from build123d import *

# Parameters (mm, degrees)
F0_W      = 228.6
F0_H      = 114.3
F1_DEPTH  = 120.65
F6_R      = 9.525
F7_DEPTH  = 38.1
F8_DEPTH  = 12.7
F10_DEPTH = 228.6
F11_R     = 9.525
F12_DEPTH = 31.75


# Not quite as in the source:
# - a pattern or mirror of a feature is missing from the dataset's text; its kind, count and spacing are read off the source's solid


with BuildPart() as f1:
    # F0 (on Top) → F1 (new body)
    with BuildSketch(Plane.XY):
        with Locations((-114.3, 57.15)):
            Rectangle(F0_W, F0_H)
    extrude(amount=F1_DEPTH)

    # F6 (on 3pt) → F7 (join, symmetric)
    with BuildSketch(Plane(origin=(-114.3, 0, 0), x_dir=(0, -1, 0), z_dir=(-1, 0, 0))):
        Polygon((-75.7497070202, 171.45), (-95.25, 120.65), (-19.05, 120.65), (-38.5502929798, 171.45), align=None)
        with Locations((-57.15, 152.4)):
            Circle(F6_R, mode=Mode.SUBTRACT)
    extrude(amount=F7_DEPTH, both=True)

    # F6 (on 3pt) → F8 (cut, symmetric)
    with BuildSketch(Plane(origin=(-114.3, 0, 0), x_dir=(0, -1, 0), z_dir=(-1, 0, 0))):
        Polygon((-75.7497070202, 171.45), (-95.25, 120.65), (-19.05, 120.65), (-38.5502929798, 171.45), align=None)
        with Locations((-57.15, 152.4)):
            Circle(F6_R, mode=Mode.SUBTRACT)
    extrude(amount=F8_DEPTH, both=True, mode=Mode.SUBTRACT)

    # F9 (on face) → F10 (cut, through all)
    with BuildSketch(Plane.YZ):
        Polygon((31.75, 120.65), (0, 120.65), (0, 76.2), align=None)
        Polygon((114.3, 120.65), (82.55, 120.65), (114.3, 76.2), align=None)
    extrude(amount=-F10_DEPTH, mode=Mode.SUBTRACT)

    # F11 (on face) → F12 (cut)
    with BuildSketch(Plane.XZ):
        with BuildLine():
            Line((-152.4, 120.65), (-133.6461139863, 87.4852331607))
            ThreePointArc((-133.6461139892, 87.4852331591), (-114.3000000002, 76.2), (-94.9538860115, 87.4852331593))
            Line((-94.9538860135, 87.4852331605), (-76.2, 120.65))
            Line((-76.2, 120.65), (-152.4, 120.65))
        make_face()
        with Locations((-114.3000000004, 98.425)):
            Circle(F11_R, mode=Mode.SUBTRACT)
    f12 = extrude(amount=-F12_DEPTH, mode=Mode.SUBTRACT)

    # F12_copies: F12 across plane
    add(f12.mirror(Plane.ZX.offset(57.15)), mode=Mode.SUBTRACT)


solid = f1.part
Can you work these out from the model? Positions are in its coordinate system, mm. A direction names the side the tool comes from. Round coordinates to 2 decimals unless told otherwise and drop trailing zeros. Write each loop counter-clockwise with the first axis right and the second up, starting at its lowest first coordinate (ties: lowest second). Pieces come first, ordered by that corner, then holes. Notation, with made-up numbers: M 14.25,26.25 L 72.25,26.25 A34 ccw 72.25,62.25 Z; hole C 8.25,-22 d6. An arc over 180 degrees is marked long. Use CSV: the item, a comma, the result in double quotes.
(1) Imagine slicing it at A-A (y = 57.15). Write out the boundary of the cut face in (x, z) (3 decimals), plus the area to 3 significant figures.
Check values:
outline,"M -228.6,0 L 0,0 L 0,120.65 L -76.2,120.65 L -76.2,142.875 L -101.6,142.875 L -101.6,120.65 L -127,120.65 L -127,142.875 L -152.4,142.875 L -152.4,120.65 L -228.6,120.65 Z; M -152.4,161.925 L -127,161.925 L -127,171.45 L -152.4,171.45 Z; M -101.6,161.925 L -76.2,161.925 L -76.2,171.45 L -101.6,171.45 Z"
area,"29,200 mm^2"
(2) We'd pull the mould along X, two halves only. Please class faces 5 (the flat face through (-89.08, 28.66, 145.69)), 6 (the flat face through (-76.2, 58, 141)), 7 (the flat face through (-115, 82.55, 109)): +X half, -X half, draft (parallel to the pull), parting line (faces both ways), or undercut.
Check values:
face 5,"draft"
face 6,"+X half"
face 7,"undercut"
(3) I need wall thicknesses on line 1 along Z through (x, y) = (-87, 57); line 2 along X through (y, z) = (38, 129.5); line 3 along X through (y, z) = (21, 94). Which ranges of each line are inside material? Lowest first, please.
Check values:
line 1,"0 to 142.88, 161.92 to 171.45"
line 2,"-152.4 to -127, -101.6 to -76.2"
line 3,"-228.6 to -137.33, -122.73 to -105.87, -91.27 to 0"
(4) Imagine slicing it at B-B (z = 152.4). Write out the boundary of the cut face in (x, y) (3 decimals), plus the area to 3 significant figures.
Check values:
outline,"M -152.4,31.238 L -127,31.238 L -127,47.625 L -152.4,47.625 Z; M -152.4,66.675 L -127,66.675 L -127,83.062 L -152.4,83.062 Z; M -101.6,31.238 L -76.2,31.238 L -76.2,47.625 L -101.6,47.625 Z; M -101.6,66.675 L -76.2,66.675 L -76.2,83.062 L -101.6,83.062 Z"
area,"1,660 mm^2"
(5) Imagine slicing it at C-C (x = -63.5). Write out the boundary of the cut face in (y, z).
Check values:
outline,"M 0,0 L 114.3,0 L 114.3,76.2 L 82.55,120.65 L 31.75,120.65 L 0,76.2 Z"
(6) On a 3-axis mill with a long thin cutter (end or side, diameter ignored), from which of +Z, -Z, +X, -X, +Y, -Y can I reach the whole of each face in a straight line? I mean faces 1 (the flat face through (-39, 58, 120.65)), 2 (the flat face through (-138.987, 89.296, 96.93)), 3 (the flat face through (-101.6, 58, 141)), 4 (the flat face through (-115, 31.75, 109)). Say none if no direction works.
Check values:
face 1,"+Z, +X, +Y, -Y"
face 2,"+Y"
face 3,"+Z, +Y, -Y"
face 4,"-Y"
(7) I'm going to push flat-ended pins straight in: pin 1 (4 mm diameter, centred on x = -78.5, y = 49.5, fed in from -Z); pin 2 (15 mm diameter, centred on y = 66.5, z = 136.5, fed in from -X); pin 3 (13.5 mm diameter, centred on x = -127, z = 106, fed in from +Y); pin 4 (15 mm diameter, centred on y = 43, z = 140, fed in from +X). Where does each tip first touch, or does it pass through?
Check values:
pin 1,"z = 0"
pin 2,"x = -152.4"
pin 3,"y = 97.21"
pin 4,"x = -76.2"
